CAD build for the part. Positions are in the model's coordinates, mm. Give positions to 0.01 mm unless a question says otherwise; leave off trailing zeros. Loops run counter-clockwise (first coordinate to the right, second up) from the corner with the lowest first, then second, coordinate; pieces in that order, holes last. Notation, with made-up numbers: (56, 47.5) - (80, 47.5) arc R21 ccw to (80, 68.5) - close; hole circle Ø2 at (-37, 52.5). An arc over 180 degrees is marked (long way). Return JSON: item names as keys, results as strings.
from build123d import *

# Parameters (mm, degrees)
ESBO_O2_W                = 150
ESBO_O2_H                = 70
ESBO_O2_R                = 1.505424276
ESBO_O2_R_2              = 1.49848088
ESBO_O2_R_3              = 1.474413832
ESBO_O2_R_4              = 1.5
ESBO_O2_R_5              = 1.55575
ESBO_O2_W_2              = 21.076348962
ESBO_O2_H_2              = 3.321026243
RESSALTO_EXTRUS_O1_DEPTH = 3
ESBO_O4_R                = 3.175
CORTE_EXTRUS_O1_DEPTH    = 3
FILETE1_R                = 7.5
ESBO_O8_R                = 6
CORTE_EXTRUS_O3_DEPTH    = 10


with BuildPart() as part:
    # Esboço2 → Ressalto-extrusão1 (new body)
    with BuildSketch(Plane(origin=(0, 0, 0), x_dir=(1, 0, 0), z_dir=(0, 1, 0))):
        with Locations((75, 35)):
            Rectangle(ESBO_O2_W, ESBO_O2_H)
        with Locations(Location((103.082572265, 55.082550604, 0), (0, 0, 270))):
            Circle(ESBO_O2_R, mode=Mode.SUBTRACT)
        with Locations(Location((69.55992433, 12.300225249, 0), (0, 0, 270))):
            Circle(ESBO_O2_R_2, mode=Mode.SUBTRACT)
        with Locations(Location((69.954401909, 55.279412058, 0), (0, 0, 270))):
            Circle(ESBO_O2_R_3, mode=Mode.SUBTRACT)
        with Locations(Location((102.570189974, 11.968678193, 0), (0, 0, 270))):
            Circle(ESBO_O2_R_4, mode=Mode.SUBTRACT)
        with Locations(Location((38.765135158, 29.268361159, 0), (0, 0, 270))):
            Circle(ESBO_O2_R_5, mode=Mode.SUBTRACT)
        with Locations(Location((54.322635158, 29.268361159, 0), (0, 0, 270))):
            Circle(ESBO_O2_R_5, mode=Mode.SUBTRACT)
        with Locations((46.559410677, 41.281799613)):
            Rectangle(ESBO_O2_W_2, ESBO_O2_H_2, mode=Mode.SUBTRACT)
    extrude(amount=RESSALTO_EXTRUS_O1_DEPTH)

    # Esboço4 → Corte-extrusão1 (cut)
    with BuildSketch(Plane(origin=(0, 3, 0), x_dir=(1, 0, 0), z_dir=(0, 1, 0))):
        with Locations(Location((10.5, 60, 0), (0, 0, 270))):
            Circle(ESBO_O4_R)
        with Locations(Location((139.5, 60, 0), (0, 0, 270))):
            Circle(ESBO_O4_R)
        with Locations(Location((139.5, 10, 0), (0, 0, 270))):
            Circle(ESBO_O4_R)
        with Locations(Location((10.5, 10, 0), (0, 0, 270))):
            Circle(ESBO_O4_R)
    extrude(amount=-CORTE_EXTRUS_O1_DEPTH, mode=Mode.SUBTRACT)

    # Filete1
    filete1_edges = [part.edges().sort_by_distance(p)[0] for p in [
        (0, 1.5, -70),
        (150, 1.5, -70),
        (150, 1.5, 0),
        (0, 1.5, 0),
    ]]
    fillet(filete1_edges, radius=FILETE1_R)

    # Esboço8 → Corte-extrusão3 (cut)
    with BuildSketch(Plane(origin=(0, 3, 0), x_dir=(1, 0, 0), z_dir=(0, 1, 0))):
        with Locations(Location((14.707477015, 35, 0), (0, 0, 270))):
            Circle(ESBO_O8_R)
        with Locations(Location((135.29252298, 35, 0), (0, 0, 270))):
            Circle(ESBO_O8_R)
    extrude(amount=-CORTE_EXTRUS_O3_DEPTH, mode=Mode.SUBTRACT)


solid = part.part
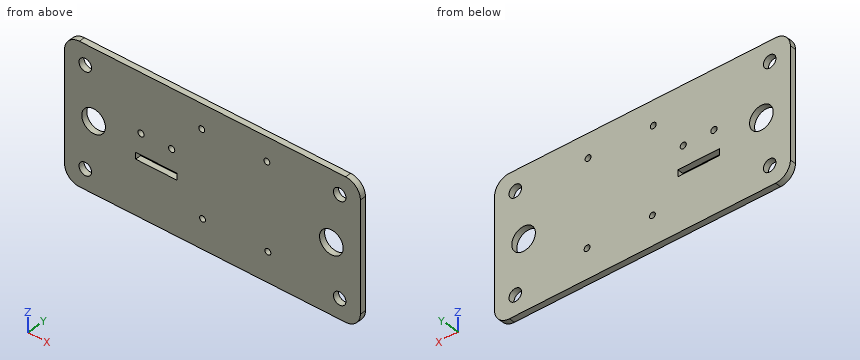
1. Cut at B-B, the plane x = 10.5. Write the cut outline in (y, z) (3 decimals).
Values follow:
{"outline": "(0, -70) - (3, -70) - (3, -63.175) - (0, -63.175) - close; (0, -56.825) - (3, -56.825) - (3, -39.278) - (0, -39.278) - close; (0, -30.722) - (3, -30.722) - (3, -13.175) - (0, -13.175) - close; (0, -6.825) - (3, -6.825) - (3, 0) - (0, 0) - close"}
2. Cut at A-A, the plane z = -35. Write the cut outline in (x, y).
Values follow:
{"outline": "(0, 0) - (8.71, 0) - (8.71, 3) - (0, 3) - close; (20.71, 0) - (129.29, 0) - (129.29, 3) - (20.71, 3) - close; (141.29, 0) - (150, 0) - (150, 3) - (141.29, 3) - close"}
3. Cut at D-D, the plane z = -60. Write the cut outline in (x, y) (3 decimals), plus the area to 3 significant figures.
Values follow:
{"outline": "(0, 0) - (7.325, 0) - (7.325, 3) - (0, 3) - close; (13.675, 0) - (136.325, 0) - (136.325, 3) - (13.675, 3) - close; (142.675, 0) - (150, 0) - (150, 3) - (142.675, 3) - close", "area": "412 mm²"}
4. Cut at C-C, the plane y = 1.8. Give the number of separate pieces and of enclosed holes in the cut face, plus the area to 3 significant figures.
Values follow:
{"separate pieces": "1", "enclosed holes": "13", "area": "9,990 mm²"}
5. Drill centre lines: probe 1 along X at (y, z) = (1.5, -60) (3 decimals); probe 2 along X at (y, z) = (1.7, -35); probe 3 along X at (y, z) = (2.4, -12). Where is each one in solid material? Low to high.
Values follow:
{"probe 1": "x = 0 to 7.325, 13.675 to 136.325, 142.675 to 150", "probe 2": "x = 0 to 8.71, 20.71 to 129.29, 141.29 to 150", "probe 3": "x = 0 to 8.03, 12.97 to 68.09, 71.03 to 101.07, 104.07 to 137.03, 141.97 to 150"}
